Part print with two shaded views. Sizes in mm from the minimum x, y, z corner. Round coordinates to 2 decimals unless told otherwise and drop trailing zeros. Loops run counter-clockwise (first coordinate to the right, second up) from the corner with the lowest first, then second, coordinate; pieces in that order, holes last. Notation, with made-up numbers: (-26, -35) - (-11, -35) arc R18 cw to (-11, -24) - close; hole circle Ø1 at (72.5, 61). An arc over 180 degrees is marked (long way). Put each result on its own line as item: value. Start each with the question number.
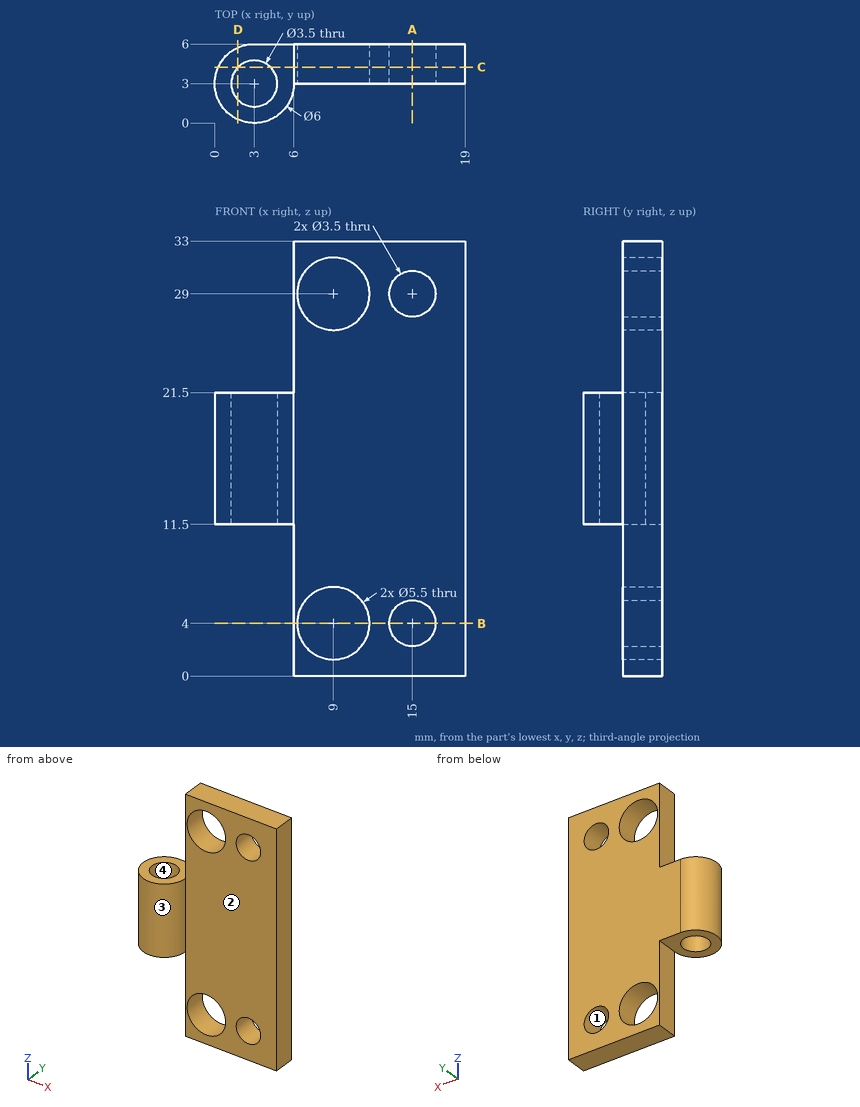
1) Slice it at C-C, the plane y = 4.25. Write the cut outline in (x, z).
2) Pull direction Y, two halves, no side cores. Call the marked faces 1, 2, 3 and 4: pulls with the +Y half, pulls with the -Y half, needs draft (parallel to the pull), parting line crosses it, or undercut.
3) Drill centre lines: line 1 (Z direction, x = 15, y = 4.8); line 2 (Z direction, x = 9, y = 4.05); line 3 (X direction, y = 3.15, z = 16). Where is each one in solid material? Low to high. Write a range as [from, to].
4) Slice it at D-D, the plane x = 1.75. Write the cut outline in (y, z).
5) Slice it at B-B, the plane z = 4. Write the cut outline in (x, y), and give its area (3 significant figures).
6) Slice it at A-A, the plane x = 15. Write the cut outline in (y, z).
7) Drop flat-ended pins along their axis: pin 1 Ø4.5 at (x, z) = (9, 4) entering from -Y; pin 2 Ø1.8 at (x, y) = (3, 2) entering from +Z; pin 3 Ø2.5 at (y, z) = (5, 28.5) entering from -X; pin 4 Ø1.8 at (x, y) = (2, 2) entering from -Z. Give the stop position or say it passes through.
Taken from the geometry:
1. outline: (0.27, 11.5) - (1.78, 11.5) - (1.78, 21.5) - (0.27, 21.5) - close; (4.22, 11.5) - (6, 11.5) - (6, 0) - (19, 0) - (19, 33) - (6, 33) - (6, 21.5) - (4.22, 21.5) - close; hole circle Ø5.5 at (9, 4); hole circle Ø5.5 at (9, 29); hole circle Ø3.5 at (15, 4); hole circle Ø3.5 at (15, 29)
2. face 1: needs draft
2. face 2: pulls with the -Y half
2. face 3: parting line crosses it
2. face 4: undercut
3. line 1: z = [0, 2.25], [5.75, 27.25], [30.75, 33]
3. line 2: z = [0, 1.25], [6.75, 26.25], [31.75, 33]
3. line 3: x = [0, 1.26], [4.74, 19]
4. outline: (0.27, 11.5) - (1.78, 11.5) - (1.78, 21.5) - (0.27, 21.5) - close; (4.22, 11.5) - (5.73, 11.5) - (5.73, 21.5) - (4.22, 21.5) - close
5. outline: (6, 3) - (6.25, 3) - (6.25, 6) - (6, 6) - close; (11.75, 3) - (13.25, 3) - (13.25, 6) - (11.75, 6) - close; (16.75, 3) - (19, 3) - (19, 6) - (16.75, 6) - close
5. area: 12.0 mm2
6. outline: (3, 0) - (6, 0) - (6, 2.25) - (3, 2.25) - close; (3, 5.75) - (6, 5.75) - (6, 27.25) - (3, 27.25) - close; (3, 30.75) - (6, 30.75) - (6, 33) - (3, 33) - close
7. pin 1: passes through
7. pin 2: stops at z = 21.5
7. pin 3: stops at x = 6
7. pin 4: stops at z = 11.5
